The model under review builds one solid part; all positions refer to its coordinate system, in mm. A direction names the side the tool comes from. Give positions to 0.01 mm unless a question says otherwise; leave off trailing zeros. Write each loop counter-clockwise with the first axis right and the second up, starting at its lowest first coordinate (ties: lowest second). Pieces come first, ordered by that corner, then holes. Notation, with made-up numbers: (79.5, 43.25) - (90.5, 43.25) arc R12 ccw to (90.5, 50.25) - close; hole circle Ø4 at (40.25, -38.5). An arc over 180 degrees is marked (long way). Write item = value, one per line.
```python
from build123d import *

# Parameters (mm, degrees)
CYLINDER004_R               = 1.35
CYLINDER004_DEPTH           = 10
CYLINDER004_PLACEMENT_ANGLE = 91
CYLINDER003_R               = 1.35
CYLINDER003_DEPTH           = 10
CYLINDER003_PITCH_ANGLE     = 90
CYLINDER002_R               = 5
CYLINDER002_DEPTH           = 20
CYLINDER002_PITCH_ANGLE     = 90
BOX_W                       = 10
BOX_H                       = 6
BOX_DEPTH                   = 22
CYLINDER001_R               = 10
CYLINDER001_DEPTH           = 154
CUT003_PITCH_ANGLE          = 90
CUT003_PLACEMENT_ANGLE      = -90


with BuildPart() as cylinder004:
    # Cylinder004 → Cylinder004 (new body)
    with BuildSketch(Plane.XY):
        Circle(CYLINDER004_R)
    extrude(amount=CYLINDER004_DEPTH)


with BuildPart() as cylinder004_1:
    # Cylinder004 placement: moved
    add(cylinder004.part.moved(Location((0, 0, 85))).rotate(Axis((0, 0, 85), (0, 1, 0)), CYLINDER004_PLACEMENT_ANGLE))


with BuildPart() as cylinder003:
    # Cylinder003 → Cylinder003 (new body)
    with BuildSketch(Plane.XY):
        Circle(CYLINDER003_R)
    extrude(amount=CYLINDER003_DEPTH)


with BuildPart() as cylinder003_1:
    # Cylinder003 pitch: moved
    add(cylinder003.part.rotate(Axis((0, 0, 0), (0, 1, 0)), CYLINDER003_PITCH_ANGLE))


with BuildPart() as cylinder003_2:
    # Cylinder003 placement: moved
    add(cylinder003_1.part.moved(Location((0, 0, 69))))


with BuildPart() as cylinder002:
    # Cylinder002 → Cylinder002 (new body)
    with BuildSketch(Plane.XY):
        Circle(CYLINDER002_R)
    extrude(amount=CYLINDER002_DEPTH)


with BuildPart() as cylinder002_1:
    # Cylinder002 pitch: moved
    add(cylinder002.part.rotate(Axis((0, 0, 0), (0, 1, 0)), CYLINDER002_PITCH_ANGLE))


with BuildPart() as cylinder002_2:
    # Cylinder002 placement: moved
    add(cylinder002_1.part.moved(Location((-10, 0, 77))))


with BuildPart() as cube:
    # Box → Box (new body)
    with BuildSketch(Plane(origin=(9.54, -3, 66), x_dir=(1, 0, 0), z_dir=(0, 0, 1))):
        with Locations((5, 3)):
            Rectangle(BOX_W, BOX_H)
    extrude(amount=BOX_DEPTH)


with BuildPart() as lever:
    # Cylinder001 → Cylinder001 (new body)
    with BuildSketch(Plane.XY):
        Circle(CYLINDER001_R)
    extrude(amount=CYLINDER001_DEPTH)

    # Cut: cut Cube
    add(cube.part, mode=Mode.SUBTRACT)

    # Cut001: cut Cylinder002
    add(cylinder002_2.part, mode=Mode.SUBTRACT)

    # Cut002: cut Cylinder003
    add(cylinder003_2.part, mode=Mode.SUBTRACT)

    # Cut003: cut Cylinder004
    add(cylinder004_1.part, mode=Mode.SUBTRACT)


with BuildPart() as lever_1:
    # Cut003 pitch: moved
    add(lever.part.rotate(Axis((0, 0, 0), (0, 1, 0)), CUT003_PITCH_ANGLE))


with BuildPart() as lever_2:
    # Cut003 placement: moved
    add(lever_1.part.moved(Location((106, 77, 0))).rotate(Axis((106, 77, 0), (0, 0, 1)), CUT003_PLACEMENT_ANGLE))


solid = lever_2.part
```
1. Take a section at C-C on y = 8. Give the boundary of the cut face in (x, z).
Findings below:
outline = (103, -9.54) - (104.65, -9.54) - (104.65, 0) - (107.35, 0) - (107.35, -9.54) - (109, -9.54) arc R10 ccw (long way) to start
2. Take a section at D-D on z = -8. Count the separate pieces of the cut face and the enclosed holes in it, and give its area (3 significant figures).
Findings below:
separate_pieces = 1
enclosed_holes = 3
area = 1,760 mm²
3. For line 1 (Y direction, x = 105.5, z = -6); line 2 (Y direction, x = 108, z = -8); line 3 (X direction, y = 8, z = -6.5), list the stretches that pass through material, from the lowest coordinate up. Write a range as from..to.
Findings below:
line_1 = -77..-9.15, -6.64..-4.97, 4.97..6.75, 9.25..77
line_2 = -77..-4.58, 4.58..77
line_3 = 98.4..104.65, 107.35..113.6
4. Machinability: for faces 1 (the cylindrical face through (104.8, 8.62, -4.7)), 2 (the cylindrical face through (110.957, -0.651, 0.367)), 3 (the flat face through (104.6, 6.8, -9.54)), which of the approach directions +Z, -Z, +X, -X, +Y, -Y give a long, thin tool a straight path to every point of the face, cutting with its end or side? Answer none if there is none.
Findings below:
face_1 = -Z
face_2 = +Z, -Z
face_3 = -Z, +X, -X
5. Insertion check: P1, Ø1, axis at x = 102.5, y = -42.5, coming from the +Z side; P2, Ø3, axis at x = 105.5, y = 8, coming from the -Z side; P3, Ø5, axis at x = 112.5, y = 59.5, coming from the -Z side; P4, Ø6, axis at x = 106, y = 0, coming from the +Z side. Each pin has a flat end and moves straight along its axis. Give the tip position at first contact, or say it passes through.
Findings below:
P1 = 9.54
P2 = -9.54
P3 = -9.17
P4 = through
6. Take a section at B-B on z = 8. Give the boundary of the cut face in (x, y).
Findings below:
outline = (100, -77) - (112, -77) - (112, 77) - (100, 77) - close; hole circle Ø10 at (106, 0)
7. Take a section at A-A on x = 106. Give the boundary of the cut face in (y, z).
Findings below:
outline = (-77, -10) - (-11, -10) - (-11, -9.54) - (-9.18, -9.54) - (-9.35, -0.02) - (-6.65, 0.02) - (-6.48, -9.54) - (-5, -9.54) - (-5, 10) - (-77, 10) - close; (5, -9.54) - (6.65, -9.54) - (6.65, 0) - (9.35, 0) - (9.35, -9.54) - (11, -9.54) - (11, -10) - (77, -10) - (77, 10) - (5, 10) - close
8. Draft analysis for pull direction Y (two halves, no side actions). For faces 4 (the flat face through (106, -77, 0)), 5 (the flat face through (106, 77, 0)), 6 (the cylindrical face through (104.8, -7.3, -4.7)), state which applies: +Y half, -Y half, draft (parallel to the pull), parting line (faces both ways), or undercut.
Findings below:
face_4 = -Y half
face_5 = +Y half
face_6 = undercut
